from build123d import *

# Parameters (mm, degrees)
F0_R     = 63.5
F1_DEPTH = 19.05
F2_DEPTH = 9.398
F4_DEPTH = 15.875


with BuildPart() as f1:
    # F0 (on Front) → F1 (new body)
    with BuildSketch(Plane.XZ):
        Circle(F0_R)
        Polygon((-49.285696, 31.858407), (45.167994, 38.940311), (-9.641714, -55.992887), align=None, mode=Mode.SUBTRACT)
    extrude(amount=F1_DEPTH)

    # F0 (on Front) → F2 (join)
    with BuildSketch(Plane.XZ):
        Polygon((-9.641714, -55.992887), (45.167994, 38.940311), (-49.285696, 31.858407), align=None)
    extrude(amount=F2_DEPTH)

    # F3 (on Top) → F4 (join, symmetric)
    with BuildSketch(Plane.XY):
        with BuildLine():
            Line((7.331135, 0), (53.051135, 0))
            Line((53.051135, 0), (53.051135, 45.72))
            Line((53.051135, 45.72), (42.891135, 45.72))
            Line((42.891135, 45.72), (42.891135, 38.676579))
            ThreePointArc((42.891135, 38.676579), (29.968754, 4.623022), (17.491135, 38.842048))
            Line((17.491135, 38.842048), (17.491135, 45.72))
            Line((17.491135, 45.72), (7.331135, 45.72))
            Line((7.331135, 45.72), (7.331135, 0))
        make_face()
    extrude(amount=F4_DEPTH, both=True)


solid = f1.part
Could you check a few things on this model? Use its own coordinates, in mm. A direction names the side the tool comes from. Coordinates: 2 decimals unless noted, no trailing zeros. Order: outer loops, then holes, each group sorted by start corner. A loop starts at its lowest first (then second) coordinate and runs counter-clockwise, first axis right, second up.
Q1. Please list where these lines run through material, in increasing order: L1, parallel to Z at x = 17, y = 5 (3 decimals); L2, parallel to Y at x = -14, z = 50; L3, parallel to X at y = -11, z = 16.5.
Q2. Which directions (+Z, -Z, +X, -X, +Y, -Y) give clear straight access to the entire face, cutting with the end or side of a thin tool? Please do faces 4 (the flat face through (-2.72, -14.16, 35.35)), 5 (the flat face through (30, 3, -15.875)), 6 (the flat face through (17.491, 42, 0)).
Q3. Will these pins go through, and if not, where does the flat tip stop? pin 1 (23 mm diameter, centred on x = 19, y = 24.5, fed in from -Z) (3 decimals); pin 2 (1.5 mm diameter, centred on x = 15.5, z = -48, fed in from +Y); pin 3 (3.5 mm diameter, centred on y = 43, z = -2, fed in from -X).
Q4. Suppose I cut it at D-D on y = -13. Please give me the cut outline in (x, z), and give its area (3 significant figures).
Q5. Suppose I cut it at A-A on y = 34. Please give me the cut outline in (x, z) (3 decimals).
Q6. Thinking about a two-plate mould opening in Y: for faces 1 (the flat face through (12, 45.72, 0)), 2 (the cylindrical face through (30.63, 4.63, 0.22)), 3 (the flat face through (18.15, -14.16, -7.86)), which applies, released by +Y, released by -Y, zero draft, split by the parting line, or undercut?
Q7. Suppose I cut it at C-C on z = -18. Please give me the cut outline in (x, y), and give its area (3 significant figures).
Q8. Suppose I cut it at B-B on x = 51.5. Please give me the cut outline in (y, z) (3 decimals).
Answer:
1. L1: z = -15.875 to 15.875
1. L2: y = -19.05 to 0
1. L3: x = -61.32 to -42.36, 32.21 to 61.32
2. face 4: -Y
2. face 5: -Z, +X, -X, +Y
2. face 6: +Z, -Z, +Y
3. pin 1: stops at z = -15.875
3. pin 2: stops at y = 0
3. pin 3: stops at x = 7.33
4. outline: circle Ø127 at (0, 0); hole (-49.29, 31.86) - (-9.64, -55.99) - (45.17, 38.94) - close
4. area: 8,380 mm2
5. outline: (7.331, -15.875) - (13.403, -15.875) - (13.403, 15.875) - (7.331, 15.875) - close; (46.788, -15.875) - (53.051, -15.875) - (53.051, 15.875) - (46.788, 15.875) - close
6. face 1: released by +Y
6. face 2: undercut
6. face 3: zero draft
7. outline: (-60.9, -19.05) - (-26.79, -19.05) - (-26.79, -9.4) - (12.29, -9.4) - (12.29, -19.05) - (60.9, -19.05) - (60.9, 0) - (-60.9, 0) - close
7. area: 1,940 mm2
8. outline: (-19.05, -37.148) - (0, -37.148) - (0, -15.875) - (45.72, -15.875) - (45.72, 15.875) - (0, 15.875) - (0, 37.148) - (-19.05, 37.148) - close
